Check sheet for the modelled part. Datum: model origin and axes. Units: mm. A direction names the side the tool comes from. Round coordinates to 2 decimals unless told otherwise and drop trailing zeros. Order: outer loops, then holes, each group sorted by start corner. A loop starts at its lowest first (then second) coordinate and runs counter-clockwise, first axis right, second up.
Q1. Cross-section at A-A on x = 0. Record the cut outline in (y, z).
Q2. Cross-section at C-C on z = -259. Record the cut outline in (x, y).
Q3. Set-up check for faces 4 (the flat face through (-5.5, -32.2, -250)), 5 (the flat face through (-29, 12, -302.15)), 6 (the cylindrical face through (-8.238, 37.096, -126.722)): record each of +Z, -Z, +X, -X, +Y, -Y from which the full face is reachable in a straight line by a thin tool's end or side.
Q4. Mould release check, pull along Z, two halves, no side actions. Record for faces 1 (the conical face through (-4.703, -35.818, -0.125)), 2 (the cylindrical face through (31, -9.76, -275.1)), 3 (the cylindrical face through (-4.036, -30.736, -300.844)): +Z half, -Z half, draft (parallel to the pull), parting line (faces both ways), or undercut.
Q5. Depth check by flat-ended pin: P1, Ø2, axis at x = 18, z = -51, coming from the -Y side; P2, Ø1.5, axis at x = 15, z = -234.5, coming from the -Y side; P3, Ø2, axis at y = -11.5, z = -256.5, coming from the +X side. Enter the tip coordinate at first touch or a pass-through.
Q6. Cross-section at D-D on z = -132. Record the cut outline in (x, y), then the cut area to 3 significant figures.
Q7. Scan lines: probe 1 along Z at (x, y) = (-11.5, 33); probe 2 along Z at (x, y) = (-2, -31.5); probe 3 along Z at (x, y) = (19.5, 25). Record each from-to range of solid material in increasing order.
from build123d import *

# Parameters (mm, degrees)
CHAMFER_1_SIZE = 2


with BuildPart() as part:
    # Эскиз1 → Повернуть1 (revolve)
    with BuildSketch(Plane(origin=(0, 0, 0), x_dir=(0, 0, -1), z_dir=(1, 0, 0)), mode=Mode.PRIVATE) as revolve_1_sk:
        Polygon((0, 0), (0, 38), (250, 38), (250, 32.5), (299.5, 32.5), (299.5, 31), (302.15, 31), (302.15, 32.5), (307.5, 32.5), (307.5, 0), align=None)
    revolve(revolve_1_sk.sketch.rotate(Axis((0, 0, 0), (0, 0, -1)), 90), axis=Axis((0, 0, 0), (0, 0, -1)))

    # Фаска1
    chamfer_1_edges = [part.edges().sort_by_distance(p)[0] for p in [
        (-38, 0, -250),
        (-38, 0, 0),
        (-32.5, 0, -307.5),
    ]]
    chamfer(chamfer_1_edges, length=CHAMFER_1_SIZE)


solid = part.part
Results found:
1. outline: (-38, -248) - (-36, -250) - (-32.5, -250) - (-32.5, -299.5) - (-31, -299.5) - (-31, -302.15) - (-32.5, -302.15) - (-32.5, -305.5) - (-30.5, -307.5) - (30.5, -307.5) - (32.5, -305.5) - (32.5, -302.15) - (31, -302.15) - (31, -299.5) - (32.5, -299.5) - (32.5, -250) - (36, -250) - (38, -248) - (38, -2) - (36, 0) - (-36, 0) - (-38, -2) - close
2. outline: circle Ø65 at (0, 0)
3. face 4: -Z
3. face 5: none
3. face 6: +Z, -Z
4. face 1: +Z half
4. face 2: draft
4. face 3: undercut
5. P1: stops at y = -33.99
5. P2: stops at y = -35.23
5. P3: stops at x = 30.76
6. outline: circle Ø76 at (0, 0)
6. area: 4,540 mm2
7. probe 1: z = -250 to 0
7. probe 2: z = -306.44 to -302.15, -299.5 to 0
7. probe 3: z = -306.29 to -302.15, -299.5 to 0
